Can you work these out from the model? Positions are in its coordinate system, mm. A direction names the side the tool comes from. Round coordinates to 2 decimals unless told otherwise and drop trailing zeros. Loops run counter-clockwise (first coordinate to the right, second up) from the corner with the lowest first, then second, coordinate; pieces in that order, holes last.
from build123d import *

# Parameters (mm, degrees)
SKETCH1_W           = 558.8
SKETCH1_H           = 304.8
BOSS_EXTRUDE1_DEPTH = 12.7
SKETCH2_W           = 304.8
SKETCH2_H           = 152.4
CUT_EXTRUDE1_DEPTH  = 12.7
SKETCH4_R           = 10.287
CUT_EXTRUDE2_DEPTH  = 12.7


with BuildPart() as part:
    # Sketch1 → Boss-Extrude1 (new body)
    with BuildSketch(Plane(origin=(0, 0, 0), x_dir=(1, 0, 0), z_dir=(0, 1, 0))):
        with Locations((219.899775418, -105.5355758)):
            Rectangle(SKETCH1_W, SKETCH1_H)
    extrude(amount=BOSS_EXTRUDE1_DEPTH)

    # Sketch2 → Cut-Extrude1 (cut)
    with BuildSketch(Plane(origin=(0, 12.7, 0), x_dir=(1, 0, 0), z_dir=(0, 1, 0))):
        with Locations((219.899775418, -105.5355758)):
            Rectangle(SKETCH2_W, SKETCH2_H)
    extrude(amount=-CUT_EXTRUDE1_DEPTH, mode=Mode.SUBTRACT)

    # Sketch4 → Cut-Extrude2 (cut)
    with BuildSketch(Plane(origin=(0, 12.7, 0), x_dir=(1, 0, 0), z_dir=(0, 1, 0))):
        with Locations((54.799775418, 8.7644242)):
            Circle(SKETCH4_R)
        with Locations((384.999775418, 8.7644242)):
            Circle(SKETCH4_R)
        with Locations((54.799775418, -219.8355758)):
            Circle(SKETCH4_R)
        with Locations((384.999775418, -219.8355758)):
            Circle(SKETCH4_R)
    extrude(amount=-CUT_EXTRUDE2_DEPTH, mode=Mode.SUBTRACT)


solid = part.part
(1) If we mould it in two halves opening along X, with no side actions, what happens to faces 1 (the flat face through (216, 0, 2)), 2 (the flat face through (499.3, 6, 108)), 3 (the flat face through (218, 6, 29.336))? For each: released by +X, released by -X, zero draft, split by the parting line, or undercut.
Worked answers:
face 1: zero draft
face 2: released by +X
face 3: undercut
(2) If we section it at D-D, the plane y = 9: List the corners of the cut face in (x, z) for me.
Worked answers:
outline: (-59.5, -46.86) - (499.3, -46.86) - (499.3, 257.94) - (-59.5, 257.94) - close; hole circle Ø20.57 at (54.8, -8.76); hole circle Ø20.57 at (54.8, 219.84); hole (67.5, 29.34) - (372.3, 29.34) - (372.3, 181.74) - (67.5, 181.74) - close; hole circle Ø20.57 at (385, -8.76); hole circle Ø20.57 at (385, 219.84)
(3) If we section it at A-A, the plane z = 76.5: List the corners of the cut face in (x, y) for me, then the cut area to 3 significant figures.
Worked answers:
outline: (-59.5, 0) - (67.5, 0) - (67.5, 12.7) - (-59.5, 12.7) - close; (372.3, 0) - (499.3, 0) - (499.3, 12.7) - (372.3, 12.7) - close
area: 3,230 mm2
(4) If I drill on line 1 (Z direction, x = 266, y = 7.75); line 2 (X direction, y = 8.5, z = 104); line 3 (Z direction, x = 54.5, y = 10.5), over which ranges is the centre line in solid material (lowest first)?
Worked answers:
line 1: z = -46.86 to 29.34, 181.74 to 257.94
line 2: x = -59.5 to 67.5, 372.3 to 499.3
line 3: z = -46.86 to -19.05, 1.52 to 209.55, 230.12 to 257.94
(5) For faces 4 (the flat face through (218, 6, 181.736)), 5 (the flat face through (216, 6, 257.936)), which set-ups out of +Z, -Z, +X, -X, +Y, -Y let a thin tool reach every point of the face, with its end or its side?
Worked answers:
face 4: +Y, -Y
face 5: +Z, +X, -X, +Y, -Y
(6) If we section it at B-B, the plane x = 313: List the corners of the cut face in (y, z) for me, then the cut area to 3 significant figures.
Worked answers:
outline: (0, -46.86) - (12.7, -46.86) - (12.7, 29.34) - (0, 29.34) - close; (0, 181.74) - (12.7, 181.74) - (12.7, 257.94) - (0, 257.94) - close
area: 1,940 mm2
(7) If we section it at C-C, the plane x = 57: List the corners of the cut face in (y, z) for me.
Worked answers:
outline: (0, -46.86) - (12.7, -46.86) - (12.7, -18.81) - (0, -18.81) - close; (0, 1.28) - (12.7, 1.28) - (12.7, 209.79) - (0, 209.79) - close; (0, 229.88) - (12.7, 229.88) - (12.7, 257.94) - (0, 257.94) - close
